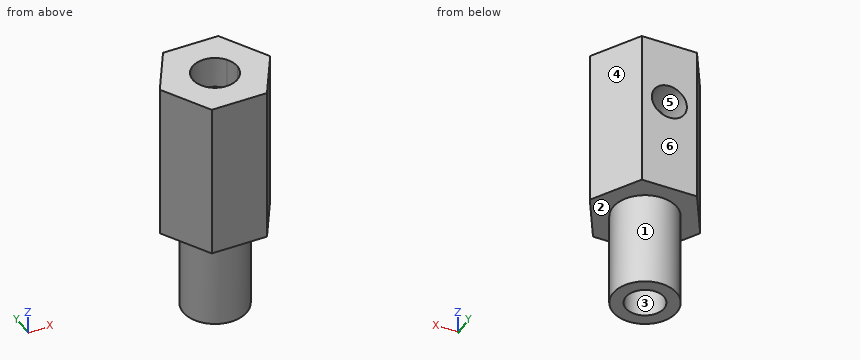
from build123d import *

# Parameters (mm, degrees)
BOSS_EXTRUDE1_DEPTH = 25.4
CUT_EXTRUDE1_DEPTH  = 8.89
SKETCH2_3_R         = 1.778
CUT_EXTRUDE2_DEPTH  = 2.54
SKETCH6_R           = 1.524
CUT_EXTRUDE3_DEPTH  = 16.51
SKETCH7_R           = 1.397
CUT_EXTRUDE4_DEPTH  = 3.81
SKETCH8_W           = 12.797374265
SKETCH8_H           = 12.133936035
CUT_EXTRUDE5_DEPTH  = 5.08
SKETCH9_R           = 5.447820482
SKETCH9_R_2         = 2.54
CUT_EXTRUDE6_DEPTH  = 7.62


with BuildPart() as part:
    # Sketch1 → Boss-Extrude1 (new body)
    with BuildSketch(Plane.XY):
        Polygon((2.199704526, 3.81), (-2.199704526, 3.81), (-4.399409051, 0), (-2.199704526, -3.81), (2.199704526, -3.81), (4.399409051, 0), align=None)
    extrude(amount=BOSS_EXTRUDE1_DEPTH)

    # Sketch2 → Cut-Extrude1 (cut)
    with BuildSketch(Plane.XY.offset(25.4)):
        with BuildLine():
            Line((1.459118912, 1.016), (-1.459118912, 1.016))
            ThreePointArc((-1.459118912, 1.016), (-0.532433364, -1.69640759), (1.778, 0))
            ThreePointArc((1.778, 0), (1.69640759, 0.532433364), (1.459118912, 1.016))
        make_face()
    extrude(amount=-CUT_EXTRUDE1_DEPTH, mode=Mode.SUBTRACT)

    # Sketch2<3> → Cut-Extrude2 (cut)
    with BuildSketch(Plane.XY.offset(25.4)):
        Circle(SKETCH2_3_R)
    extrude(amount=-CUT_EXTRUDE2_DEPTH, mode=Mode.SUBTRACT)

    # Sketch6 → Cut-Extrude3 (cut)
    with BuildSketch(Plane(origin=(0, 0, 0), x_dir=(-1, 0, 0), z_dir=(0, 0, -1))):
        Circle(SKETCH6_R)
    extrude(amount=-CUT_EXTRUDE3_DEPTH, mode=Mode.SUBTRACT)

    # Sketch7 → Cut-Extrude4 (cut)
    with BuildSketch(Plane(origin=(0, 3.81, 0), x_dir=(1, 0, 0), z_dir=(0, 1, 0))):
        with Locations((0, -20.32)):
            Circle(SKETCH7_R)
    extrude(amount=-CUT_EXTRUDE4_DEPTH, mode=Mode.SUBTRACT)

    # Sketch8 → Cut-Extrude5 (cut)
    with BuildSketch(Plane(origin=(0, 0, 0), x_dir=(-1, 0, 0), z_dir=(0, 0, -1))):
        with Locations((-0.392825268, 0.110181057)):
            Rectangle(SKETCH8_W, SKETCH8_H)
    extrude(amount=-CUT_EXTRUDE5_DEPTH, mode=Mode.SUBTRACT)

    # Sketch9 → Cut-Extrude6 (cut)
    with BuildSketch(Plane(origin=(0, 0, 5.08), x_dir=(-1, 0, 0), z_dir=(0, 0, -1))):
        Circle(SKETCH9_R)
        Circle(SKETCH9_R_2, mode=Mode.SUBTRACT)
    extrude(amount=-CUT_EXTRUDE6_DEPTH, mode=Mode.SUBTRACT)


solid = part.part
Here's how the part is built. I have some questions about the finished solid (model axes, mm). Face numbers are marked on the shaded views. A direction names the side the tool comes from. Round coordinates to 2 decimals unless told otherwise and drop trailing zeros. Order: outer loops, then holes, each group sorted by start corner. A loop starts at its lowest first (then second) coordinate and runs counter-clockwise, first axis right, second up. Notation, with made-up numbers: M 14.5,-33.75 L 48.5,-33.75 A16 ccw 48.5,-8.75 Z; hole C -23.75,-36 d5. An arc over 180 degrees is marked long. Return JSON: item names as keys, results as strings. Group by question number.
1. I'm going to push flat-ended pins straight in: pin 1 Ø2.5 at (x, y) = (0, 0) entering from -Z; pin 2 Ø3 at (x, z) = (0.5, 10.5) entering from -Y; pin 3 Ø2 at (y, z) = (0.5, 22) entering from -X. Where does each tip first touch, or does it pass through?
2. Please list where these lines run through material, in increasing order: probe 1 along Y at (x, z) = (0, 11.5); probe 2 along Z at (x, y) = (0, 2.9); probe 3 along Z at (x, y) = (0.25, -3.5).
3. If we section it at A-A on z = 17: List the corners of the cut face in (x, y) for me.
4. If we section it at C-C on y = -1: List the corners of the cut face in (x, z) for me.
5. If we section it at D-D on z = 20.32: List the corners of the cut face in (x, y) for me.
6. On a 3-axis mill with a long thin cutter (end or side, diameter ignored), from which of +Z, -Z, +X, -X, +Y, -Y can I reach the whole of each face in a straight line? I mean the marked faces 5 and 6. Say none if no direction works.
7. If we mould it in two halves opening along Y, with no side actions, what happens to the marked faces 1, 2, 3 and 4? For each: pulls with the +Y half, pulls with the -Y half, needs draft (parallel to the pull), parting line crosses it, or undercut.
8. If we section it at B-B on x = 0: List the corners of the cut face in (y, z) for me, then the cut area to 3 significant figures.
Reply:
{
 "1": {"pin 1": "z = 16.51", "pin 2": "y = -2.54", "pin 3": "x = -4.4"},
 "2": {"probe 1": "-2.54 to -1.52, 1.52 to 2.54", "probe 2": "12.7 to 18.92, 21.72 to 25.4", "probe 3": "12.7 to 25.4"},
 "3": {"outline": "M -4.4,0 L -2.2,-3.81 L 2.2,-3.81 L 4.4,0 L 2.2,3.81 L -2.2,3.81 Z; hole M -1.46,1.02 A1.78 ccw long 1.46,1.02 Z"},
 "4": {"outline": "M -3.82,12.7 L -2.33,12.7 L -2.33,5.08 L -1.15,5.08 L -1.15,16.51 L -1.47,16.51 L -1.47,25.4 L -3.82,25.4 Z; M 1.15,5.08 L 2.33,5.08 L 2.33,12.7 L 3.82,12.7 L 3.82,25.4 L 1.47,25.4 L 1.47,16.51 L 1.15,16.51 Z"},
 "5": {"outline": "M -4.4,0 L -2.2,-3.81 L 2.2,-3.81 L 4.4,0 L 2.2,3.81 L 1.4,3.81 L 1.4,1.02 L 1.46,1.02 A1.78 cw long -1.46,1.02 L -1.4,1.02 L -1.4,3.81 L -2.2,3.81 Z"},
 "6": {"face 5": "+Y", "face 6": "+Z, -Z, +X, -X, +Y"},
 "7": {"face 1": "parting line crosses it", "face 2": "needs draft", "face 3": "undercut", "face 4": "pulls with the +Y half"},
 "8": {"outline": "M -3.81,12.7 L -2.54,12.7 L -2.54,5.08 L -1.52,5.08 L -1.52,16.51 L -1.78,16.51 L -1.78,25.4 L -3.81,25.4 Z; M 1.02,16.51 L 1.52,16.51 L 1.52,5.08 L 2.54,5.08 L 2.54,12.7 L 3.81,12.7 L 3.81,18.92 L 1.02,18.92 Z; M 1.02,21.72 L 3.81,21.72 L 3.81,25.4 L 1.78,25.4 L 1.78,22.86 L 1.02,22.86 Z", "area": "66.1 mm^2"}
}
